```python
from build123d import *

# Parameters (mm, degrees)
F0_W     = 152.112037
F0_H     = 151.181682
F1_DEPTH = 76.708
F2_T     = -2.54
F3_W     = 6.279856
F3_H     = 5.814679
F4_DEPTH = 161.798
F6_W     = 7.675372
F6_H     = 6.745033
F5_W     = 6.047272
F5_H     = 6.51244
F7_W     = 8.605727
F7_H     = 5.349502
F8_DEPTH = 177.292


with BuildPart() as f1:
    # F0 (on Front) → F1 (new body)
    with BuildSketch(Plane.XZ):
        with Locations((-0.232585, 0.465177)):
            Rectangle(F0_W, F0_H)
    extrude(amount=F1_DEPTH)

    # F2
    f2_openings = [f1.faces().sort_by_distance(p)[0] for p in [
        (-0.232585, -76.708, 0.465177),
    ]]
    offset(amount=F2_T, openings=f2_openings)

    # F3 (on face) → F4 (join)
    with BuildSketch(Plane.XZ.offset(2.54)):
        with Locations((-72.960392, 72.916087)):
            Rectangle(F3_W, F3_H)
    extrude(amount=F4_DEPTH)

    # F6 (on face) + F5 (on face) + F7 (on face) → F8 (join)
    with BuildSketch(Plane.XZ.offset(2.54)):
        with Locations((71.708854, -70.822808)):
            Rectangle(F6_W, F6_H)
    with BuildSketch(Plane.XZ.offset(2.54)):
        with Locations((-73.076684, -71.869444)):
            Rectangle(F5_W, F5_H)
    with BuildSketch(Plane.XZ.offset(2.54)):
        with Locations((71.47627, 73.613852)):
            Rectangle(F7_W, F7_H)
    extrude(amount=F8_DEPTH)


solid = f1.part
```
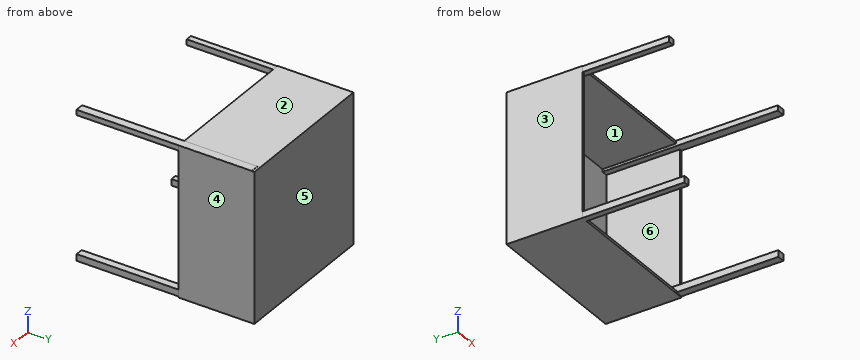
Geometry check sheet. Reference: the model listing, model coordinates, mm. Face numbers are marked on the shaded views. A direction names the side the tool comes from. Round coordinates to 2 decimals unless told otherwise and drop trailing zeros. Write each loop counter-clockwise with the first axis right and the second up, starting at its lowest first coordinate (ties: lowest second). Pieces come first, ordered by that corner, then holes. Notation, with made-up numbers: (-21, -36.75) -> (-17, -36.75) arc R7 cw to (-17, -26.75) -> close; hole circle Ø10 at (69.25, -5). An arc over 180 degrees is marked (long way). Put each result on its own line as item: value.
1) Depth check by flat-ended pin: P1, Ø1.5, axis at x = 1, z = -57, coming from the -Y side; P2, Ø7.5, axis at y = -125.5, z = -69.5, coming from the -X side; P3, Ø23, axis at x = 24, y = -50, coming from the +Z side. Enter the tip coordinate at first touch or a pass-through.
Recorded:
P1: stops at y = -2.54
P2: stops at x = -76.1
P3: stops at z = 76.06
2) Cross-section at C-C, the plane y = -31.5. Enter the section's corners in (x, z).
Recorded:
outline: (-76.29, -75.13) -> (75.82, -75.13) -> (75.82, 76.06) -> (75.78, 76.06) -> (75.78, 76.29) -> (67.17, 76.29) -> (67.17, 76.06) -> (-76.29, 76.06) -> close; hole (-73.75, -68.61) -> (-70.05, -68.61) -> (-70.05, -72.59) -> (67.87, -72.59) -> (67.87, -67.45) -> (73.28, -67.45) -> (73.28, 70.94) -> (67.17, 70.94) -> (67.17, 73.52) -> (-69.82, 73.52) -> (-69.82, 70.01) -> (-73.75, 70.01) -> close
3) Cross-section at B-B, the plane x = -22. Enter the section's corners in (y, z).
Recorded:
outline: (-76.71, -75.13) -> (0, -75.13) -> (0, 76.06) -> (-76.71, 76.06) -> (-76.71, 73.52) -> (-2.54, 73.52) -> (-2.54, -72.59) -> (-76.71, -72.59) -> close
4) Thickness scan on probe 1 along Z at (x, y) = (-43, -15.5); probe 2 along X at (y, z) = (-69, 57); probe 3 along Y at (x, z) = (43, -0.5). Record the ranges inside material, lowest first. Write a range as from..to.
Recorded:
probe 1: z = -75.13..-72.59, 73.52..76.06
probe 2: x = -76.29..-73.75, 73.28..75.82
probe 3: y = -2.54..0
5) Cross-section at D-D, the plane z = 5. Enter the section's corners in (x, y), plus the area to 3 significant figures.
Recorded:
outline: (-76.29, -76.71) -> (-73.75, -76.71) -> (-73.75, -2.54) -> (73.28, -2.54) -> (73.28, -76.71) -> (75.82, -76.71) -> (75.82, 0) -> (-76.29, 0) -> close
area: 763 mm2
6) Release check for a two-part mould opening along X. For the marked faces 1, 2, 3 and 4 record: pulls with the +X half, pulls with the -X half, needs draft (parallel to the pull), parting line crosses it, or undercut.
Recorded:
face 1: undercut
face 2: needs draft
face 3: pulls with the -X half
face 4: pulls with the +X half
7) Access from +Z, -Z, +X, -X, +Y, -Y to the whole of each face (thin tool, end or side, straight path). Record for the marked faces 5 and 6.
Recorded:
face 5: +Z, -Z, +X, -X, +Y
face 6: -Y
8) Cross-section at A-A, the plane y = -86.5. Enter the section's corners in (x, z), plus the area to 3 significant figures.
Recorded:
outline: (-76.1, -75.13) -> (-70.05, -75.13) -> (-70.05, -68.61) -> (-76.1, -68.61) -> close; (-76.1, 70.01) -> (-69.82, 70.01) -> (-69.82, 75.82) -> (-76.1, 75.82) -> close; (67.17, 70.94) -> (75.78, 70.94) -> (75.78, 76.29) -> (67.17, 76.29) -> close; (67.87, -74.2) -> (75.55, -74.2) -> (75.55, -67.45) -> (67.87, -67.45) -> close
area: 174 mm2
